Can you work these out from the model? Positions are in its coordinate system, mm. A direction names the side the tool comes from. Give positions to 0.01 mm unless a question says otherwise; leave off trailing zeros. Order: outer loops, then holes, each group sorted by start corner. A loop starts at its lowest first (then second) coordinate and runs counter-clockwise, first axis right, second up.
Autodesk Inventor part; units mm, degrees
ref_plane "YZ Plane" through (0, 0, 0) normal (1, 0, 0) x (0, 1, 0)
ref_plane "XZ Plane" through (0, 0, 0) normal (0, 1, 0) x (-1, 0, 0)
ref_plane "XY Plane" through (0, 0, 0) normal (0, 0, 1) x (1, 0, 0)
sketch "Sketch1" plane through (0, 0, 0) normal (0, 1, 0) x (-1, 0, 0)
  line L0 (66.675, 127) -> (-66.675, 127)
  line L1 (-66.675, 127) -> (-66.675, -127)
  line L2 (-66.675, -127) -> (66.675, -127)
  line L3 (66.675, -127) -> (66.675, 127)
  point P0 (0, 0)
  dimension "d0" = 66.675
  dimension "d1" = 133.35
  dimension "d2" = 254
  dimension "d3" = 127
extrude "Extrusion1" add sketch "Sketch1" along normal blind 5.9944
sketch "Sketch2" plane through (0, 5.9944, 0) normal (0, 1, 0) x (1, 0, 0)
  line L0 (-66.675, -127) -> (-66.675, 127)
  line L1 (-66.675, 127) -> (66.675, 127)
  line L2 (66.675, 127) -> (66.675, -127)
  line L3 (66.675, -127) -> (-66.675, -127)
  circle A0 centre (-46.675, -107) radius 1.905
  line L4 (-66.675, -127) -> (66.675, -127)
  line L5 (0, -127) -> (0, 127)
  line L6 (-66.675, 0) -> (66.675, 0)
  circle A1 centre (-46.675, 107) radius 1.905
  circle A2 centre (46.675, -107) radius 1.905
  circle A3 centre (46.675, 107) radius 1.905
  point P0 (0, 0)
  dimension "d6" = 20
  dimension "d7" = 20
  dimension "d8" = 3.81
extrude "Extrusion2" cut sketch "Sketch2" against normal blind 5.9944 contours A0 | A1 | A2 | A3
sketch "Sketch3" plane through (0, 5.9944, 0) normal (0, 1, 0) x (1, 0, 0)
  circle A0 centre (-46.675, -107) radius 1.905
  circle A1 centre (46.675, -107) radius 1.905
  circle A2 centre (46.675, 107) radius 1.905
  circle A3 centre (-46.675, 107) radius 1.905
  line L0 (-66.675, -127) -> (-66.675, 127)
  line L1 (-66.675, 127) -> (66.675, 127)
  line L2 (66.675, 127) -> (66.675, -127)
  line L3 (66.675, -127) -> (-66.675, -127)
  line L4 (-66.675, 0) -> (66.675, 0)
  line L5 (66.675, 127) -> (-66.675, 127)
  line L6 (0, 127) -> (0, -127)
  line L7 (-66.675, -127) -> (66.675, -127)
  circle A4 centre (-38.1, -38.1) radius 1.905
  circle A5 centre (-38.1, 38.1) radius 1.905
  circle A6 centre (38.1, -38.1) radius 1.905
  circle A7 centre (38.1, 38.1) radius 1.905
  point P0 (0, 0)
  dimension "d11" = 3.81
  dimension "d12" = 38.1
  dimension "d13" = 38.1
extrude "Extrusion3" cut sketch "Sketch3" against normal blind 5.9944 contours A4 | A5 | A6 | A7
sketch "Sketch4" plane through (0, 5.9944, 0) normal (0, 1, 0) x (1, 0, 0)
  circle A0 centre (-38.1, 38.1) radius 1.905
  circle A1 centre (38.1, -38.1) radius 1.905
  circle A2 centre (38.1, 38.1) radius 1.905
  circle A3 centre (-38.1, -38.1) radius 1.905
  circle A4 centre (-46.675, -107) radius 1.905
  circle A5 centre (46.675, -107) radius 1.905
  circle A6 centre (46.675, 107) radius 1.905
  circle A7 centre (-46.675, 107) radius 1.905
  line L0 (-66.675, -127) -> (-66.675, 127)
  line L1 (-66.675, 127) -> (66.675, 127)
  line L2 (66.675, 127) -> (66.675, -127)
  line L3 (66.675, -127) -> (-66.675, -127)
  line L4 (-22.225, -127) -> (22.225, -127)
  line L5 (22.225, -127) -> (22.225, -81.28)
  line L6 (22.225, -81.28) -> (-22.225, -81.28)
  line L7 (-22.225, -81.28) -> (-22.225, -127)
  line L8 (0, -127) -> (0, 0)
  dimension "d16" = 22.225
  dimension "d17" = 22.225
  dimension "d18" = 45.72
extrude "Extrusion4" cut sketch "Sketch4" against normal blind 5.9944 contours L7 L6 L8 L3 | L8 L6 L5 L3
properties part number "TopBase"
1) We'd pull the mould along X, two halves only. Please class faces 1 (the face through (66.675, 3, 2)), 2 (the face through (1, 3, -127)), 3 (the face through (-22.225, 3, 104)): +X half, -X half, draft (parallel to the pull), parting line (faces both ways), or undercut.
2) Suppose I cut it at A-A (y = 4). Give the number of separate pieces and of enclosed holes in the cut face, and give its area (3 significant figures).
3) Suppose I cut it at B-B (z = 94). Please give me the cut outline in (x, y) (3 decimals), and give its area (3 significant figures).
4) I'm going to push flat-ended pins straight in: pin 1 Ø3.5 at (x, z) = (46.675, -107) entering from -Y; pin 2 Ø3 at (x, y) = (-5, 4) entering from +Z. Where does each tip first touch, or does it pass through?
5) Which directions (+Z, -Z, +X, -X, +Y, -Y) give clear straight access to the entire face, cutting with the end or side of a thin tool? Please do faces 4 (the face through (22.225, 3, 104)), 5 (the face through (1, 5.994, 2)).
6) If I drill on line 1 (Z direction, x = 38.1, y = 1.3) (3 decimals); line 2 (X direction, y = 0.25, z = 38) (3 decimals); line 3 (Z direction, x = -46, y = 3.15), over which ranges is the centre line in solid material (lowest first)?
Results:
1. face 1: +X half
1. face 2: draft
1. face 3: undercut
2. separate pieces: 1
2. enclosed holes: 8
2. area: 31,700 mm2
3. outline: (-66.675, 0) - (-22.225, 0) - (-22.225, 5.994) - (-66.675, 5.994) - close; (22.225, 0) - (66.675, 0) - (66.675, 5.994) - (22.225, 5.994) - close
3. area: 533 mm2
4. pin 1: passes through
4. pin 2: stops at z = 81.28
5. face 4: +Z, +Y, -Y
5. face 5: +Z, -Z, +X, -X, +Y
6. line 1: z = -127 to -40.005, -36.195 to 36.195, 40.005 to 127
6. line 2: x = -66.675 to -40.002, -36.198 to 36.198, 40.002 to 66.675
6. line 3: z = -127 to -108.78, -105.22 to 105.22, 108.78 to 127
